Geometry check sheet. Reference: the model listing, model coordinates, mm. Coordinates: 2 decimals unless noted, no trailing zeros. Order: outer loops, then holes, each group sorted by start corner. A loop starts at its lowest first (then second) coordinate and runs counter-clockwise, first axis right, second up. Notation, with made-up numbers: (-3.75, -21) -> (10.25, -21) arc R11 ccw to (10.25, -13) -> close; hole circle Ø4 at (29, -35.75). An arc over 180 degrees is marked (long way). Answer in a Markdown table with one row per item. Add a question column.
Autodesk Inventor part; units mm, degrees
ref_plane "YZ Plane" through (0, 0, 0) normal (1, 0, 0) x (0, 1, 0)
ref_plane "XZ Plane" through (0, 0, 0) normal (0, 1, 0) x (-1, 0, 0)
ref_plane "XY Plane" through (0, 0, 0) normal (0, 0, 1) x (1, 0, 0)
sketch "Sketch1" plane through (0, 0, 0) normal (1, 0, 0) x (0, 1, 0)
  circle A0 centre (0, 0) radius 26.2509
  circle A1 centre (0, 0) radius 30.1625
  dimension "d0" = 52.5018
  dimension "d1" = 3.9116
extrude "Extrusion1" add sketch "Sketch1" along normal mid plane 339
sketch "Sketch2" plane through (0, 0, 0) normal (0, 1, 0) x (1, 0, 0)
  circle A0 centre (-131.4, 0) radius 5.25
  line L0 (-169.5, -26.2509) -> (-169.5, 26.2509)
  point P0 (0, 0)
  dimension "d4" = 10.5
  dimension "d5" = 38.1
extrude "Extrusion2" cut sketch "Sketch2" along normal through all both and the other way through all
sketch "Sketch3" plane through (0, 0, 0) normal (0, 1, 0) x (-1, 0, 0)
  circle A0 centre (144.2, 0) radius 2.625
  circle A1 centre (118.8, 0) radius 2.6358
  line L0 (0, 0) -> (162.823, 0) construction
  line L1 (131.5, 0) -> (131.5, -16.0563) construction
  line L2 (169.5, 26.2509) -> (169.5, -26.2509) construction
  dimension "d8" = 5.25
  dimension "d9" = 25.4
  dimension "d10" = 38
extrude "Extrusion3" cut sketch "Sketch3" along normal through all both and the other way through all
properties part number "Arm Segment 2" material "PVC-Piping"
(1) Cross-section at C-C (x = 23). Enter the section's corners in (y, z) (1 decimal).
(2) Scan lines: line 1 along X through (y, z) = (27.6, 0) (3 decimals); line 2 along Z through (x, y) = (66.5, 0.5); line 3 along Z through (x, y) = (-101.5, 6.5). Record each from-to range of solid material in increasing order.
(3) Mould release check, pull along Y, two halves, no side actions. Record for faces 1 (the face through (-2.373, -30.133, -1.326)), 2 (the face through (-146.7, -28.1, 0.8)), 3 (the face through (2.373, -3.417, 26.028)): +Y half, -Y half, draft (parallel to the pull), parting line (faces both ways), or undercut.
(4) Go/stop test with flat-tipped pins: P1, Ø12, axis at x = -114, z = -18, coming from the +Y side; P2, Ø4, axis at x = -144.2, z = 0, coming from the +Y side; P3, Ø1, axis at x = -73, y = 9.5, coming from the +Z side; P4, Ø5, axis at x = -44, z = 14.5, coming from the -Y side. Record where each tip stops, or that it passes through.
(5) Cross-section at A-A (y = 0). Enter the section's corners in (x, z).
(6) Cross-section at B-B (z = 13.5). Enter the section's corners in (x, y).
Checks:
| question | item | result |
|---|---|---|
| 1 | outline | circle Ø60.3 at (0, 0); hole circle Ø52.5 at (0, 0) |
| 2 | line 1 | -169.5 to -146.825, -141.575 to -136.65, -126.15 to -121.436, -116.164 to 169.5 |
| 2 | line 2 | -30.16 to -26.25, 26.25 to 30.16 |
| 2 | line 3 | -29.45 to -25.43, 25.43 to 29.45 |
| 3 | face 1 | parting line |
| 3 | face 2 | draft |
| 3 | face 3 | undercut |
| 4 | P1 | y = 27.67 |
| 4 | P2 | through |
| 4 | P3 | z = 28.79 |
| 4 | P4 | y = -27.67 |
| 5 | outline | (-169.5, -30.16) -> (169.5, -30.16) -> (169.5, -26.25) -> (-169.5, -26.25) -> close; (-169.5, 26.25) -> (169.5, 26.25) -> (169.5, 30.16) -> (-169.5, 30.16) -> close |
| 6 | outline | (-169.5, -26.97) -> (169.5, -26.97) -> (169.5, -22.51) -> (-169.5, -22.51) -> close; (-169.5, 22.51) -> (169.5, 22.51) -> (169.5, 26.97) -> (-169.5, 26.97) -> close |
